Autodesk Inventor part; units mm, degrees
ref_plane "YZ Plane" through (0, 0, 0) normal (1, 0, 0) x (0, 1, 0)
ref_plane "XZ Plane" through (0, 0, 0) normal (0, 1, 0) x (-1, 0, 0)
ref_plane "XY Plane" through (0, 0, 0) normal (0, 0, 1) x (1, 0, 0)
sketch "Sketch1" plane through (0, 0, 0) normal (0, 1, 0) x (-1, 0, 0)
  line L0 (0, 0) -> (29.5, 0)
  line L1 (29.5, -15) -> (29.5, -102.5)
  line L2 (0.8775, -104.5) -> (0, -104.5)
  line L3 (0, -102.5) -> (0, -15)
  line L4 (0, -93.5) -> (0, -102)
  line L5 (0, -43.5) -> (0, -56.5)
  line L6 (29.5, 0) -> (0, 0)
  line L7 (0, 0) -> (0, -15)
  line L8 (29.5, -15) -> (29.5, 0)
  arc A0 (27.5, -104.5) -> (29.5, -102.5) centre (27.5, -102.5) ccw
  line L9 (27.5, -104.5) -> (12, -104.5)
  line L10 (27.5, -104.5) -> (12, -104.5)
  line L11 (0, -104.5) -> (0.8775, -104.5)
  line L12 (12, -104.5) -> (12, -106)
  line L13 (12, -106) -> (4, -106)
  line L14 (0, -102) -> (0, -104.5)
  arc A1 (0, -102) -> (4, -106) centre (4, -102) ccw
  point P0 (29.5, -104.5)
  point P1 (11, -104.5)
  point P2 (0, -102)
  point P3 (0, -106)
  dimension "d0" = 29.5
  dimension "d1" = 104.5
  dimension "d7" = 15
  dimension "d8" = 2
  dimension "d40" = 12
  dimension "d41" = 1.5
  dimension "d42" = 4
extrude "Extrusion1" add sketch "Sketch1" along normal blind 5 contours L0 L8 L1 A0 L9 L12 L13 A1 L3 L7
sketch "Sketch2" plane through (0, 5, 0) normal (0, 1, 0) x (1, 0, 0)
  line L0 (-9.5, -6.918) -> (-9.5, 116.4057) construction
  line L1 (0, 0) -> (0, 102) construction
  line L2 (-29.5, 102.5) -> (-29.5, 0)
  point P0 (-9.5, 84)
  point P1 (-9.5, 46)
  point P2 (-29.5, 16)
  point P3 (0, 16)
  point P4 (0, 102.5)
  point P5 (0, 104.5)
  dimension "d13" = 46
  dimension "d14" = 84
  dimension "d23" = 20
hole "Hole1" at (-9.5, 5, -84) at (-9.5, 5, -46) direction (0, -1, 0) diameter 3.2 end through all
sketch "Sketch3" plane through (0, 5, 0) normal (0, 1, 0) x (1, 0, 0)
  line L0 (-29.5, 0) -> (0, 0)
  line L1 (-29.5, 0) -> (-14.5, 0)
  line L2 (-14.5, 0) -> (-14.5, 16)
  line L3 (-18.5, 20) -> (-29.5, 20)
  line L4 (-29.5, 20) -> (-29.5, 0)
  arc A0 (-14.5, 16) -> (-18.5, 20) centre (-18.5, 16) ccw
  point P0 (-14.5, 20)
  dimension "d26" = 15
  dimension "d27" = 20
  dimension "d28" = 4
extrude "Extrusion2" cut sketch "Sketch3" against normal through all
sketch "Sketch4" plane through (0, 5, 0) normal (0, 1, 0) x (1, 0, 0)
  line L0 (0, 0) -> (0, 102)
  line L1 (-4, 106) -> (-12, 106)
  point P0 (-7.5, 101.5)
  dimension "d31" = 7.5
  dimension "d43" = 4.5
hole "Hole2" at (-7.5, 5, -101.5) direction (0, -1, 0) diameter 3.8 end through all
fillet "Fillet1" radius 2 1 edges at (-12, 2.5, -106)
properties part number "Upper slide"
Can you work these out from the model? Positions are in its coordinate system, mm. A direction names the side the tool comes from. Round coordinates to 2 decimals unless told otherwise and drop trailing zeros. Order: outer loops, then holes, each group sorted by start corner. A loop starts at its lowest first (then second) coordinate and runs counter-clockwise, first axis right, second up. Notation, with made-up numbers: (-1.5, 13.5) -> (27.5, 13.5) arc R28 ccw to (27.5, 34.5) -> close; hole circle Ø10 at (59.5, 73). An arc over 180 degrees is marked (long way). Return JSON: item names as keys, results as strings. Group by question number.
1. We'd pull the mould along Z, two halves only. Please class faces 1 (the face through (-15, 0, -52)), 2 (the face through (-7.58, 2.46, -103.4)), 3 (the face through (-1.203, 2.465, -104.859)), 4 (the face through (-7, 2, 0)): released by +Z, released by -Z, zero draft, split by the parting line, or undercut.
2. If we section it at A-A, the plane z = -46: Write out the boundary of the cut face in (x, y).
3. If we section it at C-C, the plane z = -10: Write out the boundary of the cut face in (x, y), then the cut area to 3 significant figures.
4. If we section it at D-D, the plane x = -24.25: Write out the boundary of the cut face in (y, z), then the cut area to 4 significant figures.
5. I need wall thicknesses on line 1 (Z direction, x = -9.5, y = 1.6); line 2 (X direction, y = 3.75, z = -46); line 3 (X direction, y = 1.8, z = -101.5). Which ranges of each line are inside material? Lowest first, please. Write a range as [from, to].
6. Will these pins go through, and if not, where does the flat tip stop? pin 1 (1.5 mm diameter, centred on x = -24.5, y = 3.5, fed in from +Z); pin 2 (5 mm diameter, centred on x = -9.5, z = -46, fed in from +Y); pin 3 (2.5 mm diameter, centred on y = 3.5, z = -6.5, fed in from -X).
7. If we section it at B-B, the plane y = 3.35: Write out the boundary of the cut face in (x, z), then the cut area to 3 significant figures.
8. Which directions (+Z, -Z, +X, -X, +Y, -Y) give clear straight access to the entire face, cutting with the end or side of a thin tool? Please do faces 5 (the face through (-14.5, 3, -8)), 6 (the face through (-20, 2, -104.5)), 7 (the face through (0, 2, -50)).
Output values:
{
 "1": {"face 1": "zero draft", "face 2": "undercut", "face 3": "released by -Z", "face 4": "released by +Z"},
 "2": {"outline": "(-29.5, 0) -> (-11.1, 0) -> (-11.1, 5) -> (-29.5, 5) -> close; (-7.9, 0) -> (0, 0) -> (0, 5) -> (-7.9, 5) -> close"},
 "3": {"outline": "(-14.5, 0) -> (0, 0) -> (0, 5) -> (-14.5, 5) -> close", "area": "72.5 mm²"},
 "4": {"outline": "(0, -104.5) -> (5, -104.5) -> (5, -20) -> (0, -20) -> close", "area": "422.5 mm²"},
 "5": {"line 1": "[-106, -85.6], [-82.4, -47.6], [-44.4, 0]", "line 2": "[-29.5, -11.1], [-7.9, 0]", "line 3": "[-29.5, -9.4], [-5.6, 0]"},
 "6": {"pin 1": "z = -20", "pin 2": "y = 5", "pin 3": "x = -14.5"},
 "7": {"outline": "(-29.5, -102.5) arc R2 ccw to (-27.5, -104.5) -> (-12, -104.5) arc R2 ccw to (-10.06, -106) -> (-4, -106) arc R4 ccw to (0, -102) -> (0, 0) -> (-14.5, 0) -> (-14.5, -16) arc R4 cw to (-18.5, -20) -> (-29.5, -20) -> close; hole circle Ø3.2 at (-9.5, -84); hole circle Ø3.2 at (-9.5, -46); hole circle Ø3.8 at (-7.5, -101.5)", "area": "2,770 mm²"},
 "8": {"face 5": "+Z, -X, +Y, -Y", "face 6": "-Z, -X, +Y, -Y", "face 7": "+Z, -Z, +X, +Y, -Y"}
}
